Solid Edge part; units mm, degrees
sketch "Sketch1" plane through (0, 0, 0) normal (0, -1, 0) x (1, 0, 0)
  circle A0 centre (0, 0) radius 12
extrude "Protrusion1" add sketch "Sketch1" along normal blind 10.8
chamfer "Chamfer_1" distance 1.7 angle 45 2 edges at (-12, -10.8, 0) (-12, 0, 0)
sketch "Sketch2" plane through (0, -10.8, 0) normal (0, -1, 0) x (1, 0, 0)
  line L0 (0, 12) -> (-10.3923, 6)
  line L1 (-10.3923, 6) -> (-13.1704, 9.9939)
  line L2 (-13.1704, 9.9939) -> (-1.4905, 14.5877)
  line L3 (-1.4905, 14.5877) -> (0, 12)
extrude "ExtrudedCutout_1" cut sketch "Sketch2" against normal blind 81.3692
pattern_circular "Pattern1" count 6 over 360 about axis through (0, -10.8, 0) along (0, -1, 0) of "ExtrudedCutout_1"
hole "Hole_1" at (0, -10.8, 0) direction (0, 1, 0) diameter 10.106 end up to next
chamfer "Chamfer_2" distance 1 angle 45 2 edges at (-5.053, -10.8, 0) (0, 0, -5.053)
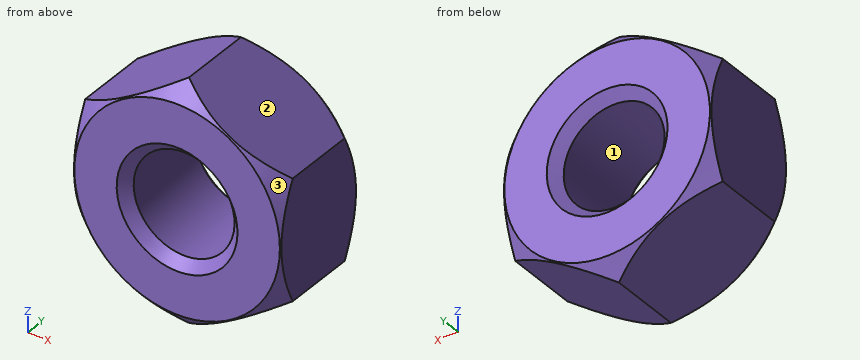
Check sheet for the modelled part. Datum: model origin and axes. Units: mm. Face numbers are marked on the shaded views. Round coordinates to 2 decimals unless told otherwise and drop trailing zeros. Order: outer loops, then holes, each group sorted by start corner. A loop starts at its lowest first (then second) coordinate and runs counter-clockwise, first axis right, second up. Notation, with made-up numbers: M 33,8.25 L 54,8.25 A6 cw 54,12.25 Z; hole C -22,60 d4. An arc over 180 degrees is marked long. Answer in a Markdown table with one row per item.
(1) Material ranges on line 1 along X through (y, z) = (-3.25, 0); line 2 along X through (y, z) = (-4, -3.5); line 3 along Z through (x, y) = (-2.75, -6), recorded low to high. Write a range as from..to.
Findings:
| item | result |
|---|---|
| line 1 | x = -10.39..-5.05, 5.05..10.39 |
| line 2 | x = -10.39..-3.64, 3.64..10.39 |
| line 3 | z = -10.41..-4.24, 4.24..10.41 |
(2) Gauge pin test, flat ends, axial feed: pin 1 (4 mm diameter, centred on x = -8, y = -9, fed in from -Z); pin 2 (3 mm diameter, centred on x = -2.5, y = -5, fed in from -Z); pin 3 (3 mm diameter, centred on x = 5.5, z = -3, fed in from +Y). Record the tip position at first contact, or that the pin passes through.
Findings:
| item | result |
|---|---|
| pin 1 | stops at z = -8.54 |
| pin 2 | stops at z = -11.42 |
| pin 3 | stops at y = 0 |
(3) Section check A-A on z = 0. Record the boundary of the cut face in (x, y), plus the area to 3 significant figures.
Findings:
| item | result |
|---|---|
| outline | M -10.39,-10.71 L -10.3,-10.8 L -6.05,-10.8 L -5.05,-9.8 L -5.05,-1 L -6.05,0 L -10.3,0 L -10.39,-0.09 Z; M 5.05,-9.8 L 6.05,-10.8 L 10.3,-10.8 L 10.39,-10.71 L 10.39,-0.09 L 10.3,0 L 6.05,0 L 5.05,-1 Z |
| area | 113 mm^2 |
(4) Draft check along Z on the marked faces 1, 2 and 3. Enter one of: +Z half, -Z half, draft (parallel to the pull), parting line (faces both ways), or undercut.
Findings:
| item | result |
|---|---|
| face 1 | undercut |
| face 2 | +Z half |
| face 3 | parting line |
(5) Section check B-B on y = -7.5. Record the boundary of the cut face in (x, z).
Findings:
| item | result |
|---|---|
| outline | M -10.39,-6 L 0,-12 L 10.39,-6 L 10.39,6 L 0,12 L -10.39,6 Z; hole C 0,0 d10.11 |
